Work out the finished part from the listing and answer in its coordinate system (mm). Round coordinates to 2 decimals unless told otherwise and drop trailing zeros. Order: outer loops, then holes, each group sorted by start corner. A loop starts at its lowest first (then second) coordinate and runs counter-clockwise, first axis right, second up.
from build123d import *

# Parameters (mm, degrees)
F0_W     = 152.4
F0_H     = 191.2747
F1_DEPTH = 19.05
F3_D     = 6.5278
F6_D     = 6.7564


with BuildPart() as f1:
    # F0 (on Top) → F1 (new body)
    with BuildSketch(Plane.XY):
        Rectangle(F0_W, F0_H)
    extrude(amount=F1_DEPTH)

    # F3 (through all)
    with Locations(Plane.XY.offset(19.05)):
        with Locations((-30.48, -86.11235), (-10.16, -86.11235), (10.16, -86.11235), (30.48, -86.11235), (-66.675, 48.01235), (-66.675, 86.11235), (66.675, 86.11235), (66.675, 48.01235), (-45.72, 10.68705), (-45.72, -22.61235), (-15.24, -22.61235), (-15.24, 10.68705), (15.24, 10.68705), (15.24, -22.61235), (45.72, -22.61235), (45.72, 10.68705)):
            Hole(F3_D / 2)

    # F6 (through all)
    with Locations(Plane.XY.offset(19.05)):
        with Locations((0, -48.8890202521), (-21.43125, -48.8890202521), (21.43125, -48.8890202521)):
            Hole(F6_D / 2)


solid = f1.part
Item 1: Find section C-C (x = 10). Write down the section's boundary in (y, z), plus the area to 3 significant figures.
Item 2: For a pull along Y with two mould halves and no side action, classify faces 1 (the face through (-1, -95.637, 9)), 2 (the face through (76.2, -1, 9)), 3 (the face through (0.732, -52.187, 9.392)) as released by +Y, released by -Y, zero draft, split by the parting line, or undercut.
Item 3: Find section D-D (x = 30.48). Write down the section's boundary in (y, z), plus the area to 3 significant figures.
Item 4: Find section A-A (x = -45.72). Write down the section's boundary in (y, z), plus the area to 3 significant figures.
Item 5: Find section B-B (z = 4). State how many separate pieces and enclosed holes the cut face has, plus the area to 3 significant figures.
Item 6: Find the intervals of material crossed by line 1 along Y through (x, z) = (-45.72, 5.75); line 2 along Y through (x, z) = (44.5, 2); line 3 along X through (y, z) = (84.5, 4.25), in increasing order.
Item 7: Given pin 1 (6 mm diameter, centred on x = -30.48, y = -86.11, fed in from -Z), flat-ended and moving along its own axis, determine where the tip first touches the part or whether it passes through.
Model answer:
1. outline: (-95.64, 0) - (-89.37, 0) - (-89.37, 19.05) - (-95.64, 19.05) - close; (-82.85, 0) - (95.64, 0) - (95.64, 19.05) - (-82.85, 19.05) - close
1. area: 3,520 mm2
2. face 1: released by -Y
2. face 2: zero draft
2. face 3: undercut
3. outline: (-95.64, 0) - (-89.38, 0) - (-89.38, 19.05) - (-95.64, 19.05) - close; (-82.85, 0) - (95.64, 0) - (95.64, 19.05) - (-82.85, 19.05) - close
3. area: 3,520 mm2
4. outline: (-95.64, 0) - (-25.88, 0) - (-25.88, 19.05) - (-95.64, 19.05) - close; (-19.35, 0) - (7.42, 0) - (7.42, 19.05) - (-19.35, 19.05) - close; (13.95, 0) - (95.64, 0) - (95.64, 19.05) - (13.95, 19.05) - close
4. area: 3,400 mm2
5. separate pieces: 1
5. enclosed holes: 19
5. area: 28,500 mm2
6. line 1: y = -95.64 to -25.88, -19.35 to 7.42, 13.95 to 95.64
6. line 2: y = -95.64 to -25.64, -19.59 to 7.66, 13.71 to 95.64
6. line 3: x = -76.2 to -69.51, -63.84 to 63.84, 69.51 to 76.2
7. pin 1: passes through
